The listing builds one solid part. Answer for the finished solid, in the listing's coordinates (mm). Give positions to 0.01 mm unless a question says otherwise; leave off trailing zeros. Write each loop counter-clockwise with the first axis right and the second up, starting at its lowest first coordinate (ties: lowest second). Pieces come first, ordered by that corner, then holes. Notation, with made-up numbers: M -13.75,19 L 9.25,19 A13 cw 9.25,30 Z; hole C -9.75,-23.75 d4. An arc over 180 degrees is marked long. Answer as a JSON object with one key per item and string values.
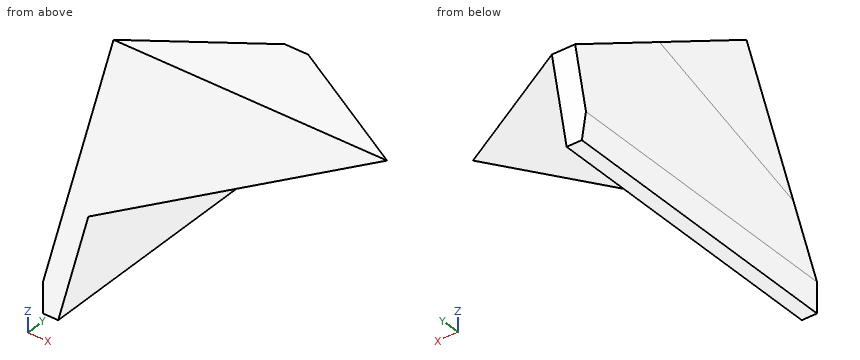
```python
from build123d import *

# Parameters (mm, degrees)
PAD_DEPTH       = 50
POCKET_DEPTH    = 5
PAD001_DEPTH    = 50
POCKET002_DEPTH = 80
POCKET003_DEPTH = 100


with BuildPart() as part:
    # Sketch → Pad (new body)
    with BuildSketch(Plane.XZ):
        Polygon((0, 5), (12.940952, 53.296291), (15.440949, 48.296292), (2.5, 0), (0, 0), align=None)
    extrude(amount=PAD_DEPTH)

    # Sketch001 (on Face3 of Pad) → Pocket (cut)
    with BuildSketch(Plane(origin=(-1.25, 0, 0.334936), x_dir=(-0.258819, 0, -0.965926), z_dir=(-0.965926, 0, 0.258819))):
        Polygon((-54.829629, 0), (-54.829629, 50), (-19.829629, 50), (-49.652199, 0), align=None)
    extrude(amount=-POCKET_DEPTH, mode=Mode.SUBTRACT)

    # Sketch002 → Pad001 (join)
    with BuildSketch(Plane.XZ):
        Polygon((11.600935, 48.295278), (3.882286, 19.488887), (7.464816, 18.528951), (56.600935, 18.528951), (56.600935, 48.295278), align=None)
    extrude(amount=PAD001_DEPTH)

    # Sketch005 → Pocket002 (cut)
    with BuildSketch(Plane.YZ):
        Polygon((0, 48.295278), (0, 0), (-3.267149, 18.528951), (-50, 48.295278), align=None)
    extrude(amount=POCKET002_DEPTH, mode=Mode.SUBTRACT)

    # Sketch007 → Pocket003 (cut)
    with BuildSketch(Plane.XZ):
        Polygon((7.464816, 18.528951), (56.600935, 18.528951), (56.600935, 48.295278), align=None)
    extrude(amount=POCKET003_DEPTH, mode=Mode.SUBTRACT)


solid = part.part
```
1. Flat-ended cylindrical pins translate along their axes: pin 1 (6 mm diameter, centred on y = -19, z = 12.5, fed in from -X); pin 2 (2 mm diameter, centred on y = -13, z = 25.5, fed in from -X) (3 decimals); pin 3 (10 mm diameter, centred on x = 13.5, z = 32, fed in from +Y). Find the tip coordinate at first contact, or state that the pin passes through.
Verdict:
{"pin 1": "stops at x = 1.21", "pin 2": "stops at x = 5.225", "pin 3": "stops at y = -16.57"}
2. A cutting plane is placed at C-C, the plane z = 39. Give the vertices of the cut face in (x, y), plus the area to 3 significant figures.
Verdict:
{"outline": "M 9.11,-50 L 41.26,-50 L 41.26,-35.41 L 9.11,-35.41 Z", "area": "469 mm2"}
3. A cutting plane is placed at A-A, the plane y = -43. Give the vertices of the cut face in (x, z).
Verdict:
{"outline": "M 0,0 L 2.5,0 L 7.46,18.53 L 49.24,43.84 L 10.41,43.84 L 0,5 Z"}
4. A cutting plane is placed at D-D, the plane y = -28. Give the vertices of the cut face in (x, z), plus the area to 3 significant figures.
Verdict:
{"outline": "M 0,0 L 2.5,0 L 7.46,18.53 L 33.47,34.28 L 7.85,34.28 L 0,5 Z", "area": "300 mm2"}
5. A cutting plane is placed at B-B, the plane x = 16. Give the vertices of the cut face in (y, z), plus the area to 3 significant figures.
Verdict:
{"outline": "M -50,23.7 L -11.38,23.7 L -50,48.3 Z", "area": "475 mm2"}
6. Consider line 1 along X through (y, z) = (-44.5, 5); line 2 along Z through (x, y) = (27, -34); line 3 along X through (y, z) = (-42.5, 10). Determine where each line is inside the solid, lowest interval first.
Verdict:
{"line 1": "x = 0 to 3.84", "line 2": "z = 30.36 to 38.1", "line 3": "x = 1.34 to 5.18"}
